Work out the finished part from the listing and answer in its coordinate system (mm). Face numbers are marked on the shaded views. Give positions to 0.01 mm unless a question says otherwise; leave off trailing zeros. Order: outer loops, then holes, each group sorted by start corner. A loop starts at its lowest first (then second) coordinate and runs counter-clockwise, first axis right, second up. Notation, with made-up numbers: (72, 69) - (99, 69) arc R23 cw to (99, 80) - close; hole circle Ø9 at (13, 13). An arc over 180 degrees is marked (long way). Put each result on its own line as item: value.
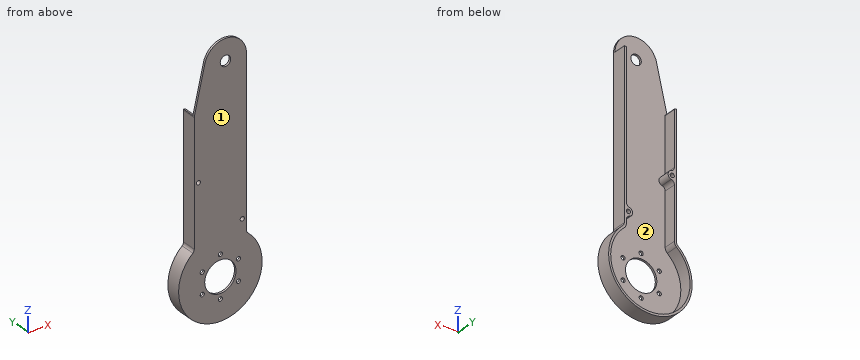
```python
from build123d import *

# Parameters (mm, degrees)
SKETCH1_R           = 1.27
SKETCH1_R_2         = 3.175
SKETCH1_R_3         = 9.525
BOSS_EXTRUDE1_DEPTH = 8.89
FILLET1_R           = 2.54
SHELL2_START        = 1.27
SHELL2_OUTLINE_R    = 3.175
SHELL2_OUTLINE_R_2  = 1.27
SHELL2_OUTLINE_R_3  = 9.525
SHELL2_DEPTH        = 7.62
FILLET2_R           = 2.54


# Read off the part's stored shape, not the designer's step: Shell2
with BuildPart() as part:
    # Sketch1 → Boss-Extrude1 (new body)
    with BuildSketch(Plane(origin=(0, 0, 0), x_dir=(1, 0, 0), z_dir=(0, 1, 0))):
        with BuildLine():
            Line((-15.875, -19.827868645), (-15.875, -96.027868645))
            Line((-15.875, -96.027868645), (-9.362396438, -124.297332186))
            ThreePointArc((-9.362396438, -124.297332186), (4.537150087, -134.127868645), (15.875, -121.427868645))
            Line((15.875, -121.427868645), (15.875, -96.027868645))
            Line((15.875, -96.027868645), (15.875, -19.827868645))
            ThreePointArc((15.875, -19.827868645), (0, 25.4), (-15.875, -19.827868645))
        make_face()
        with Locations(Location((0, 12.7, 0), (0, 0, 270))):
            Circle(SKETCH1_R, mode=Mode.SUBTRACT)
        with Locations(Location((10.998522628, 6.35, 0), (0, 0, 270))):
            Circle(SKETCH1_R, mode=Mode.SUBTRACT)
        with Locations(Location((10.998522628, -6.35, 0), (0, 0, 270))):
            Circle(SKETCH1_R, mode=Mode.SUBTRACT)
        with Locations(Location((0, -12.7, 0), (0, 0, 270))):
            Circle(SKETCH1_R, mode=Mode.SUBTRACT)
        with Locations(Location((-10.998522628, -6.35, 0), (0, 0, 270))):
            Circle(SKETCH1_R, mode=Mode.SUBTRACT)
        with Locations(Location((-10.998522628, 6.35, 0), (0, 0, 270))):
            Circle(SKETCH1_R, mode=Mode.SUBTRACT)
        with Locations(Location((3.093174395, -121.427868645, 0), (0, 0, 270))):
            Circle(SKETCH1_R_2, mode=Mode.SUBTRACT)
        with Locations(Location((-13.335, -57.927868645, 0), (0, 0, 270))):
            Circle(SKETCH1_R, mode=Mode.SUBTRACT)
        with Locations(Location((13.335, -28.25059986, 0), (0, 0, 270))):
            Circle(SKETCH1_R, mode=Mode.SUBTRACT)
        with Locations(Location((0, 0, 0), (0, 0, 270))):
            Circle(SKETCH1_R_3, mode=Mode.SUBTRACT)
    extrude(amount=BOSS_EXTRUDE1_DEPTH)

    # Fillet1
    fillet1_edges = [part.edges().sort_by_distance(p)[0] for p in [
        (15.875, 4.445, 19.827868645),
        (-15.875, 4.445, 96.027868645),
        (-15.875, 4.445, 19.827868645),
    ]]
    fillet(fillet1_edges, radius=FILLET1_R)

    # Shell2 outline → Shell2 (cut)
    with BuildSketch(Plane(origin=(0, 0, 0), x_dir=(1, 0, 0), z_dir=(0, 1, 0)).offset(SHELL2_START)):
        with BuildLine():
            Line((14.605, -121.427868645), (14.605, -30.450304386))
            ThreePointArc((14.605, -30.450304386), (10.795, -28.25059986), (14.605, -26.050895335))
            Line((14.605, -26.050895335), (14.605, -21.012647977))
            ThreePointArc((14.605, -21.012647977), (14.944875395, -19.439645997), (15.903863636, -18.147286889))
            ThreePointArc((15.903863636, -18.147286889), (0, 24.13), (-15.903863636, -18.147286889))
            ThreePointArc((-15.903863636, -18.147286889), (-14.944875395, -19.439645997), (-14.605, -21.012647977))
            Line((-14.605, -21.012647977), (-14.605, -55.728164119))
            ThreePointArc((-14.605, -55.728164119), (-10.795, -57.927868645), (-14.605, -60.127573171))
            Line((-14.605, -60.127573171), (-14.605, -95.739073507))
            ThreePointArc((-14.605, -95.739073507), (-14.596869822, -95.882546684), (-14.572583382, -96.024182912))
            Line((-14.572583382, -96.024182912), (-15.810166764, -96.309292317))
            Line((-15.810166764, -96.309292317), (-9.362396438, -124.297332186))
            ThreePointArc((-9.362396438, -124.297332186), (4.537150087, -134.127868645), (15.875, -121.427868645))
            Line((15.875, -121.427868645), (14.605, -121.427868645))
        make_face()
        with Locations((3.093174395, -121.427868645)):
            Circle(SHELL2_OUTLINE_R, mode=Mode.SUBTRACT)
        with Locations((-10.998522628, -6.35)):
            Circle(SHELL2_OUTLINE_R_2, mode=Mode.SUBTRACT)
        with Locations((0, -12.7)):
            Circle(SHELL2_OUTLINE_R_2, mode=Mode.SUBTRACT)
        Circle(SHELL2_OUTLINE_R_3, mode=Mode.SUBTRACT)
        with Locations((-10.998522628, 6.35)):
            Circle(SHELL2_OUTLINE_R_2, mode=Mode.SUBTRACT)
        with Locations((0, 12.7)):
            Circle(SHELL2_OUTLINE_R_2, mode=Mode.SUBTRACT)
        with Locations((10.998522628, -6.35)):
            Circle(SHELL2_OUTLINE_R_2, mode=Mode.SUBTRACT)
        with Locations((10.998522628, 6.35)):
            Circle(SHELL2_OUTLINE_R_2, mode=Mode.SUBTRACT)
    extrude(amount=SHELL2_DEPTH, mode=Mode.SUBTRACT)

    # Fillet2
    fillet2_edges = [part.edges().sort_by_distance(p)[0] for p in [
        (14.605, 5.08, 30.450304386),
        (-14.605, 5.08, 55.728164119),
        (-14.605, 5.08, 60.127573171),
        (14.605, 5.08, 26.050895335),
    ]]
    fillet(fillet2_edges, radius=FILLET2_R)


solid = part.part
```
(1) Determine the mould class of the marked faces 1 and 2 for opening direction X: pulls with the +X half, pulls with the -X half, needs draft (parallel to the pull), parting line crosses it, or undercut.
Geometry check:
face 1: needs draft
face 2: undercut
(2) Section B-B, the plane y = 6.5 is taken. Write down the section's boundary in (x, z) (3 decimals), then the cut area to 3 significant figures.
Geometry check:
outline: (-16.741, 19.102) arc R25.4 ccw (long way) to (16.741, 19.102) arc R2.54 cw to (15.875, 21.013) - (15.875, 121.428) - (14.605, 121.428) - (14.605, 33.169) arc R2.54 cw to (12.7, 30.71) arc R2.54 ccw to (12.7, 25.791) arc R2.54 cw to (14.605, 23.332) - (14.605, 21.013) arc R3.81 ccw to (15.904, 18.147) arc R24.13 cw (long way) to (-15.904, 18.147) arc R3.81 ccw to (-14.605, 21.013) - (-14.605, 53.009) arc R2.54 cw to (-12.7, 55.469) arc R2.54 ccw to (-12.7, 60.387) arc R2.54 cw to (-14.605, 62.847) - (-14.605, 95.739) arc R1.27 cw to (-14.573, 96.024) - (-15.81, 96.309) arc R2.54 ccw to (-15.875, 95.739) - (-15.875, 21.013) arc R2.54 cw to start; hole circle Ø2.54 at (-13.335, 57.928); hole circle Ø2.54 at (13.335, 28.251)
area: 410 mm²
(3) Straight lines are drawn through the part: line 1 (X direction, y = 6.25, z = 0); line 2 (X direction, y = 0.9, z = 0) (3 decimals); line 3 (Y direction, x = 4, z = 88.5). For each, find the intervals that lie inside material, in ascending order.
Geometry check:
line 1: x = -25.4 to -24.13, 24.13 to 25.4
line 2: x = -25.4 to -9.525, 9.525 to 25.4
line 3: y = 0 to 1.27
(4) Section C-C, the plane z = 105 is taken. Write down the section's boundary in (x, y) (3 decimals).
Geometry check:
outline: (-13.808, 0) - (15.875, 0) - (15.875, 8.89) - (14.605, 8.89) - (14.605, 1.27) - (-13.808, 1.27) - close
(5) Given pin 1 (1.4 mm diameter, centred on x = 15.5, y = 6, fed in from +Z); pin 2 (1.5 mm diameter, centred on x = -13.34, z = 57.93, fed in from +Y); pin 3 (5 mm diameter, centred on x = 17.5, y = 5, fed in from -Z); pin 4 (4.5 mm diameter, centred on y = 4, z = 75, fed in from -X) (3 decimals), each flat-ended and moving along its own axis, determine where each tip first touches the part or whether it passes through.
Geometry check:
pin 1: stops at z = 121.43
pin 2: passes through
pin 3: stops at z = -20.5
pin 4: stops at x = -15.875
(6) Section A-A, the plane z = 67 is taken. Write down the section's boundary in (x, y) (3 decimals).
Geometry check:
outline: (-15.875, 0) - (15.875, 0) - (15.875, 8.89) - (14.605, 8.89) - (14.605, 1.27) - (-14.605, 1.27) - (-14.605, 8.89) - (-15.875, 8.89) - close
